Here's how the part is built. I have some questions about the finished solid (model axes, mm). Face numbers are marked on the shaded views. A direction names the side the tool comes from. Give positions to 0.01 mm unless a question says otherwise; leave off trailing zeros. Write each loop counter-clockwise with the first axis right and the second up, starting at its lowest first coordinate (ties: lowest second). Pieces come first, ordered by that corner, then holes. Notation, with made-up numbers: (9.25, 26) - (30.25, 26) arc R27 cw to (30.25, 61) - close; hole circle Ø3 at (-22, 85.5). An arc over 180 degrees is marked (long way). One line per item, written item: value. Start each with the question number.
1) I'm going to push flat-ended pins straight in: P1, Ø1.5, axis at x = 2.5, y = -0.5, coming from the -Z side; P2, Ø2, axis at x = -0.5, z = 11, coming from the -Y side; P3, Ø0.5, axis at x = 0, y = 0, coming from the -Z side; P4, Ø3, axis at y = 2, z = 5, coming from the -X side. Where does each tip first touch, or does it pass through?
2) Imagine slicing it at A-A on x = 0. Write out the boundary of the cut face in (y, z).
3) Imagine slicing it at C-C on x = 2.75. Write out the boundary of the cut face in (y, z).
4) Please list where these lines run through material, in increasing order: L1, parallel to Z at x = -0.5, y = 3.25; L2, parallel to Y at x = 0, z = 8.75; L3, parallel to Z at x = -2.75, y = 0. Write a range as [from, to].
5) On a 3-axis mill with a long thin cutter (end or side, diameter ignored), from which of +Z, -Z, +X, -X, +Y, -Y can I reach the whole of each face in a straight line? I mean the marked faces 1 and 2. Say none if no direction works.
6) Imagine slicing it at B-B on z = 4. Write out the boundary of the cut face in (x, y), plus the area to 3 significant figures.
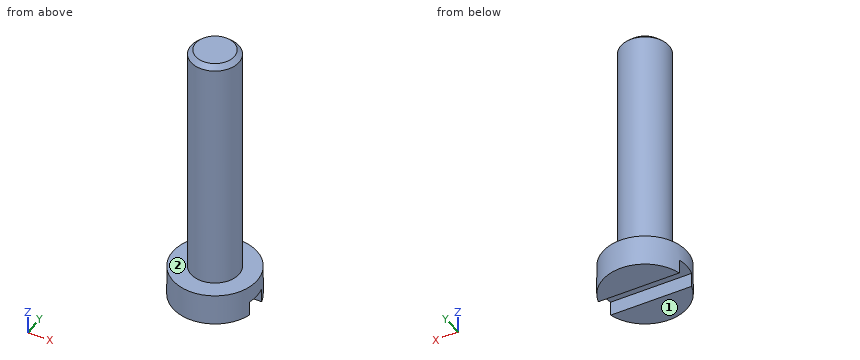
from build123d import *

# Parameters (mm, degrees)
SKETCH_1_R          = 2
EXTRUDE_1_DEPTH     = 20
SKETCH_2_R          = 3.5
EXTRUDE_2_DEPTH     = 2.6
SKETCH_3_W          = 9
SKETCH_3_H          = 1.8
CUT_EXTRUDE_1_DEPTH = 1.2
CHAMFER_1_SIZE      = 0.39


with BuildPart() as part:
    # Эскиз1 → Бобышка-Вытянуть1 (new body)
    with BuildSketch(Plane.XY):
        Circle(SKETCH_1_R)
    extrude(amount=EXTRUDE_1_DEPTH)

    # Эскиз2 → Бобышка-Вытянуть2 (add)
    with BuildSketch(Plane(origin=(0, 0, 0), x_dir=(-1, 0, 0), z_dir=(0, 0, -1))):
        Circle(SKETCH_2_R)
    extrude(amount=EXTRUDE_2_DEPTH)

    # Эскиз3 → Вырез-Вытянуть1 (cut)
    with BuildSketch(Plane(origin=(0, 0, -2.6), x_dir=(-1, 0, 0), z_dir=(0, 0, -1))):
        Rectangle(SKETCH_3_W, SKETCH_3_H)
    extrude(amount=-CUT_EXTRUDE_1_DEPTH, mode=Mode.SUBTRACT)

    # Фаска1
    chamfer_1_edges = [part.edges().sort_by_distance(p)[0] for p in [
        (-2, 0, 20),
    ]]
    chamfer(chamfer_1_edges, length=CHAMFER_1_SIZE)


solid = part.part
Numbers:
1. P1: z = -2.6
1. P2: y = -2
1. P3: z = -1.4
1. P4: x = -1.94
2. outline: (-3.5, -2.6) - (-0.9, -2.6) - (-0.9, -1.4) - (0.9, -1.4) - (0.9, -2.6) - (3.5, -2.6) - (3.5, 0) - (2, 0) - (2, 19.61) - (1.61, 20) - (-1.61, 20) - (-2, 19.61) - (-2, 0) - (-3.5, 0) - close
3. outline: (-2.17, -2.6) - (-0.9, -2.6) - (-0.9, -1.4) - (0.9, -1.4) - (0.9, -2.6) - (2.17, -2.6) - (2.17, 0) - (-2.17, 0) - close
4. L1: [-2.6, 0]
4. L2: [-2, 2]
4. L3: [-1.4, 0]
5. face 1: -Z, +X, -X, +Y, -Y
5. face 2: +Z
6. outline: circle Ø4 at (0, 0)
6. area: 12.6 mm^2
